Source: CAD feature listing. Evaluate the final solid. Frame: model axes, mm. A direction names the side the tool comes from. Coordinates: 2 decimals unless noted, no trailing zeros. Order: outer loops, then holes, each group sorted by start corner. A loop starts at its lowest first (then second) coordinate and runs counter-clockwise, first axis right, second up.
Item 1: Section C-C on y = 4. Return the cut outline in (x, z), then the cut area to 3 significant figures.
Item 2: Section A-A on y = 6. Return the cut outline in (x, z), then the cut area to 3 significant figures.
Item 3: Reachability of faces 1 (the flat face through (-4.944, 6, 7)), 2 (the flat face through (-33, 5.288, -28)), 3 (the flat face through (-14, 2, 6.446)), 4 (the flat face through (-0.944, 6, 7)) from +Z, -Z, +X, -X, +Y, -Y: full face, straight path, thin tool, end or side. Return the list, or none.
Item 4: Ray query, line 1 (X direction, y = 3.5, z = -9.5); line 2 (Z direction, x = -20, y = 3.5); line 3 (Y direction, x = -27.5, z = -25). Return the intervals inside material, ascending.
Item 5: Section B-B on x = -16. Return the cut outline in (y, z).
Item 6: Mould query, pull axis Z, two halves, no side actions, for faces 5 (the flat face through (-34.444, 5, -11)), 6 (the flat face through (-15, 5, -30.054)), 7 (the cylindrical face through (-32.09, 3.35, -27.65)), 8 (the cylindrical face through (-14.206, 0.855, 7.044)). Classes: released by +Z, released by -Z, zero draft, split by the parting line, or undercut.
Item 7: Section D-D on z = -7. Return the cut outline in (x, y), then the cut area to 3 significant figures.
Item 8: Contact query for flat-ended pins moving along their axis: P1, Ø0.8, axis at y = 6, z = -29.5, coming from the -X side; P2, Ø0.8, axis at x = 4, z = -25.5, coming from the +Y side; P3, Ø0.5, axis at y = 5, z = 7.5, coming from the +X side. Output: stop coordinate, or through.
from build123d import *

# Parameters (mm, degrees)
BOSS_EXTRUDE1_DEPTH = 7.288380162
CUT_EXTRUDE3_DEPTH  = 5.938619602
SKETCH5_W           = 8
SKETCH5_H           = 2.8
SKETCH5_W_2         = 15
SKETCH5_H_2         = 1.082982858
CUT_EXTRUDE6_DEPTH  = 4
FILLET2_R           = 3
SKETCH7_W           = 19
SKETCH7_H           = 6.03347221
CUT_EXTRUDE8_DEPTH  = 2
SKETCH8_W           = 14.334368534
SKETCH8_H           = 11.344502268
SKETCH8_W_2         = 12.278418615
SKETCH8_H_2         = 17.135054821
SKETCH8_W_3         = 15.257811301
SKETCH8_H_3         = 9.410205862
SKETCH8_W_4         = 12.235138376
SKETCH8_H_4         = 13.74281341
CUT_EXTRUDE9_DEPTH  = 2
SKETCH9_W           = 12
SKETCH9_H           = 10.54511274
CUT_EXTRUDE10_DEPTH = 2


with BuildPart() as part:
    # Sketch1 → Boss-Extrude1 (new body)
    with BuildSketch(Plane(origin=(0, 0, 0), x_dir=(1, 0, 0), z_dir=(0, 1, 0))):
        with BuildLine():
            Line((-31.444201696, 30.054028384), (2.555798304, 30.054028384))
            ThreePointArc((2.555798304, 30.054028384), (4.677118648, 29.175348727), (5.555798304, 27.054028384))
            Line((5.555798304, 27.054028384), (5.555798304, -4.945971616))
            ThreePointArc((5.555798304, -4.945971616), (4.677118648, -7.06729196), (2.555798304, -7.945971616))
            Line((2.555798304, -7.945971616), (-31.444201696, -7.945971616))
            ThreePointArc((-31.444201696, -7.945971616), (-33.565522039, -7.06729196), (-34.444201696, -4.945971616))
            Line((-34.444201696, -4.945971616), (-34.444201696, 27.054028384))
            ThreePointArc((-34.444201696, 27.054028384), (-33.565522039, 29.175348727), (-31.444201696, 30.054028384))
        make_face()
    extrude(amount=BOSS_EXTRUDE1_DEPTH)

    # Sketch2 → Cut-Extrude3 (cut)
    with BuildSketch(Plane(origin=(0, 7.288380162, 0), x_dir=(1, 0, 0), z_dir=(0, 1, 0))):
        with BuildLine():
            Line((-29.944201696, 28.554028384), (1.055798304, 28.554028384))
            ThreePointArc((1.055798304, 28.554028384), (3.177118648, 27.675348727), (4.055798304, 25.554028384))
            Line((4.055798304, 25.554028384), (4.055798304, -3.445971616))
            ThreePointArc((4.055798304, -3.445971616), (3.177118648, -5.56729196), (1.055798304, -6.445971616))
            Line((1.055798304, -6.445971616), (-29.944201696, -6.445971616))
            ThreePointArc((-29.944201696, -6.445971616), (-32.065522039, -5.56729196), (-32.944201696, -3.445971616))
            Line((-32.944201696, -3.445971616), (-32.944201696, 25.554028384))
            ThreePointArc((-32.944201696, 25.554028384), (-32.065522039, 27.675348727), (-29.944201696, 28.554028384))
        make_face()
    extrude(amount=-CUT_EXTRUDE3_DEPTH, mode=Mode.SUBTRACT)

    # Sketch5 → Cut-Extrude6 (cut)
    with BuildSketch(Plane.XY.offset(7.945971616)):
        with Locations((-14.444201696, 3.597990821)):
            Rectangle(SKETCH5_W, SKETCH5_H)
        with Locations((-14.444201696, 5.396027171)):
            Rectangle(SKETCH5_W_2, SKETCH5_H_2)
    extrude(amount=-CUT_EXTRUDE6_DEPTH, mode=Mode.SUBTRACT)

    # Fillet2
    # the kernel refuses this fillet: 3 mm, written as the material it takes off along each edge
    with BuildSketch(Plane(origin=(2.555798304, 0, 7.945971616), x_dir=(0, 0, -1), z_dir=(-1, 0, 0))) as fillet2_piece_1:
        with BuildLine():
            CenterArc((FILLET2_R, -FILLET2_R), FILLET2_R, 90, 90)
            Line((0, -FILLET2_R), (-FILLET2_R * 0.02, -FILLET2_R))
            Line((-FILLET2_R * 0.02, -FILLET2_R), (-FILLET2_R * 0.02, FILLET2_R * 0.02))
            Line((-FILLET2_R * 0.02, FILLET2_R * 0.02), (FILLET2_R, FILLET2_R * 0.02))
            Line((FILLET2_R, FILLET2_R * 0.02), (FILLET2_R, 0))
        make_face()
    extrude(amount=34, mode=Mode.SUBTRACT)
    with BuildSketch(Plane(origin=(2.555798304, 0, 4.945971616), x_dir=(1, 0, 0), z_dir=(0, 0, -1))) as fillet2_piece_2:
        with BuildLine():
            CenterArc((3 - FILLET2_R, -FILLET2_R), FILLET2_R, 0, 90)
            Line((3, -FILLET2_R), (3 + FILLET2_R * 0.02, -FILLET2_R))
            Line((3 + FILLET2_R * 0.02, -FILLET2_R), (3 + FILLET2_R * 0.02, 0))
            Line((3 + FILLET2_R * 0.02, 0), (3, FILLET2_R * 0.02))
            Line((3, FILLET2_R * 0.02), (3 - FILLET2_R, FILLET2_R * 0.02))
            Line((3 - FILLET2_R, FILLET2_R * 0.02), (3 - FILLET2_R, 0))
        make_face()
    revolve(axis=Axis((2.555798304, 0, 4.945971616), (0, -1, 0)), revolution_arc=90, mode=Mode.SUBTRACT)
    with BuildSketch(Plane(origin=(5.555798304, 0, -27.054028384), x_dir=(-1, 0, 0), z_dir=(0, 0, 1)), Plane(origin=(-34.444201696, 0, 4.945971616), x_dir=(1, 0, 0), z_dir=(0, 0, -1))) as fillet2_piece_3:
        with BuildLine():
            CenterArc((FILLET2_R, -FILLET2_R), FILLET2_R, 90, 90)
            Line((0, -FILLET2_R), (-FILLET2_R * 0.02, -FILLET2_R))
            Line((-FILLET2_R * 0.02, -FILLET2_R), (-FILLET2_R * 0.02, FILLET2_R * 0.02))
            Line((-FILLET2_R * 0.02, FILLET2_R * 0.02), (FILLET2_R, FILLET2_R * 0.02))
            Line((FILLET2_R, FILLET2_R * 0.02), (FILLET2_R, 0))
        make_face()
    extrude(amount=32, mode=Mode.SUBTRACT)
    with BuildSketch(Plane(origin=(2.555798304, 0, -27.054028384), x_dir=(0, 0, -1), z_dir=(-1, 0, 0))) as fillet2_piece_4:
        with BuildLine():
            CenterArc((3 - FILLET2_R, -FILLET2_R), FILLET2_R, 0, 90)
            Line((3 - FILLET2_R, 0), (3 - FILLET2_R, FILLET2_R * 0.02))
            Line((3 - FILLET2_R, FILLET2_R * 0.02), (3, FILLET2_R * 0.02))
            Line((3, FILLET2_R * 0.02), (3 + FILLET2_R * 0.02, 0))
            Line((3 + FILLET2_R * 0.02, 0), (3 + FILLET2_R * 0.02, -FILLET2_R))
            Line((3 + FILLET2_R * 0.02, -FILLET2_R), (3, -FILLET2_R))
        make_face()
    revolve(axis=Axis((2.555798304, 0, -27.054028384), (0, -1, 0)), revolution_arc=90, mode=Mode.SUBTRACT)
    with BuildSketch(Plane(origin=(-31.444201696, 0, -30.054028384), x_dir=(0, 1, 0), z_dir=(1, 0, 0))) as fillet2_piece_5:
        with BuildLine():
            CenterArc((FILLET2_R, FILLET2_R), FILLET2_R, 180, 90)
            Line((0, FILLET2_R), (-FILLET2_R * 0.02, FILLET2_R))
            Line((-FILLET2_R * 0.02, FILLET2_R), (-FILLET2_R * 0.02, -FILLET2_R * 0.02))
            Line((-FILLET2_R * 0.02, -FILLET2_R * 0.02), (FILLET2_R, -FILLET2_R * 0.02))
            Line((FILLET2_R, -FILLET2_R * 0.02), (FILLET2_R, 0))
        make_face()
    extrude(amount=34, mode=Mode.SUBTRACT)
    with BuildSketch(Plane(origin=(-31.444201696, 0, -27.054028384), x_dir=(-1, 0, 0), z_dir=(0, 0, 1))) as fillet2_piece_6:
        with BuildLine():
            CenterArc((3 - FILLET2_R, -FILLET2_R), FILLET2_R, 0, 90)
            Line((3 - FILLET2_R, 0), (3 - FILLET2_R, FILLET2_R * 0.02))
            Line((3 - FILLET2_R, FILLET2_R * 0.02), (3, FILLET2_R * 0.02))
            Line((3, FILLET2_R * 0.02), (3 + FILLET2_R * 0.02, 0))
            Line((3 + FILLET2_R * 0.02, 0), (3 + FILLET2_R * 0.02, -FILLET2_R))
            Line((3 + FILLET2_R * 0.02, -FILLET2_R), (3, -FILLET2_R))
        make_face()
    revolve(axis=Axis((-31.444201696, 0, -27.054028384), (0, -1, 0)), revolution_arc=90, mode=Mode.SUBTRACT)
    with BuildSketch(Plane(origin=(-31.444201696, 0, 4.945971616), x_dir=(0, 0, 1), z_dir=(1, 0, 0))) as fillet2_piece_7:
        with BuildLine():
            CenterArc((3 - FILLET2_R, -FILLET2_R), FILLET2_R, 0, 90)
            Line((3, -FILLET2_R), (3 + FILLET2_R * 0.02, -FILLET2_R))
            Line((3 + FILLET2_R * 0.02, -FILLET2_R), (3 + FILLET2_R * 0.02, 0))
            Line((3 + FILLET2_R * 0.02, 0), (3, FILLET2_R * 0.02))
            Line((3, FILLET2_R * 0.02), (3 - FILLET2_R, FILLET2_R * 0.02))
            Line((3 - FILLET2_R, FILLET2_R * 0.02), (3 - FILLET2_R, 0))
        make_face()
    revolve(axis=Axis((-31.444201696, 0, 4.945971616), (0, -1, 0)), revolution_arc=90, mode=Mode.SUBTRACT)

    # Sketch7 → Cut-Extrude8 (cut)
    with BuildSketch(Plane(origin=(0, 7.288380162, 0), x_dir=(1, 0, 0), z_dir=(0, 1, 0))):
        with Locations((-14.444201696, -7.080404366)):
            Rectangle(SKETCH7_W, SKETCH7_H)
    extrude(amount=-CUT_EXTRUDE8_DEPTH, mode=Mode.SUBTRACT)

    # Sketch8 → Cut-Extrude9 (cut)
    with BuildSketch(Plane(origin=(0, 7.288380162, 0), x_dir=(1, 0, 0), z_dir=(0, 1, 0))):
        with Locations((6.222982571, -7.11822275)):
            Rectangle(SKETCH8_W, SKETCH8_H)
        with Locations((-34.083411004, -10.013499027)):
            Rectangle(SKETCH8_W_2, SKETCH8_H_2)
        with Locations((-35.573107347, 28.259131315)):
            Rectangle(SKETCH8_W_3, SKETCH8_H_3)
        with Locations((5.173367492, 30.425435089)):
            Rectangle(SKETCH8_W_4, SKETCH8_H_4)
    extrude(amount=-CUT_EXTRUDE9_DEPTH, mode=Mode.SUBTRACT)

    # Sketch9 → Cut-Extrude10 (cut)
    with BuildSketch(Plane(origin=(0, 7.288380162, 0), x_dir=(1, 0, 0), z_dir=(0, 1, 0))):
        with Locations((-3.080143155, 28.401822491)):
            Rectangle(SKETCH9_W, SKETCH9_H)
    extrude(amount=-CUT_EXTRUDE10_DEPTH, mode=Mode.SUBTRACT)


solid = part.part
Answer list:
1. outline: (-34.44, -27.05) arc R3 ccw to (-31.44, -30.05) - (2.56, -30.05) arc R3 ccw to (5.56, -27.05) - (5.56, 4.95) arc R3 ccw to (2.56, 7.95) - (-10.44, 7.95) - (-10.44, 6.45) - (1.06, 6.45) arc R3 cw to (4.06, 3.45) - (4.06, -25.55) arc R3 cw to (1.06, -28.55) - (-29.94, -28.55) arc R3 cw to (-32.94, -25.55) - (-32.94, 3.45) arc R3 cw to (-29.94, 6.45) - (-18.44, 6.45) - (-18.44, 7.95) - (-31.44, 7.95) arc R3 ccw to (-34.44, 4.95) - close
1. area: 213 mm2
2. outline: (-34.44, -23.55) - (-32.94, -23.55) - (-32.94, 1.45) - (-34.44, 1.45) - close; (-27.94, -30.05) - (-9.08, -30.05) - (-9.08, -28.55) - (-27.94, -28.55) - close; (-27.94, 6.45) - (-23.94, 6.45) - (-23.94, 7.95) - (-27.94, 7.95) - close; (-4.94, 6.45) - (-0.94, 6.45) - (-0.94, 7.95) - (-4.94, 7.95) - close; (4.06, -23.55) - (5.56, -23.55) - (5.56, 1.45) - (4.06, 1.45) - close
2. area: 115 mm2
3. face 1: +Z, -Z, +Y
3. face 2: -Z, -X, +Y
3. face 3: +Y
3. face 4: +Z, -Z, +X, +Y
4. line 1: x = -34.44 to -32.94, 4.06 to 5.56
4. line 2: z = -30.05 to -28.55, 6.45 to 7.95
4. line 3: y = 0 to 1.35
5. outline: (0, -27.05) arc R3 ccw to (3, -30.05) - (7.29, -30.05) - (7.29, -28.55) - (1.35, -28.55) - (1.35, 6.45) - (2.2, 6.45) - (2.2, 7.84) arc R3 ccw to (0, 4.95) - close
6. face 5: zero draft
6. face 6: released by -Z
6. face 7: undercut
6. face 8: released by +Z
7. outline: (-34.44, 3) arc R3 ccw to (-31.44, 0) - (2.56, 0) arc R3 ccw to (5.56, 3) - (5.56, 7.29) - (4.06, 7.29) - (4.06, 1.35) - (-32.94, 1.35) - (-32.94, 7.29) - (-34.44, 7.29) - close
7. area: 67.9 mm2
8. P1: stops at x = -27.94
8. P2: stops at y = 5.29
8. P3: stops at x = 4.48
